Source: CAD feature listing. Evaluate the final solid. Frame: model axes, mm. Face numbers are marked on the shaded views. A direction names the side the tool comes from. Give positions to 0.01 mm unless a question says otherwise; leave off trailing zeros. Loops run counter-clockwise (first coordinate to the right, second up) from the corner with the lowest first, then second, coordinate; pieces in that order, holes last. Notation, with made-up numbers: (16, -4) -> (32, -4) arc R11 cw to (32, 17) -> close; hole circle Ø6 at (24.25, 49.5). An arc over 180 degrees is marked (long way). Answer as a JSON object with one key per item and string values. Group by question number.
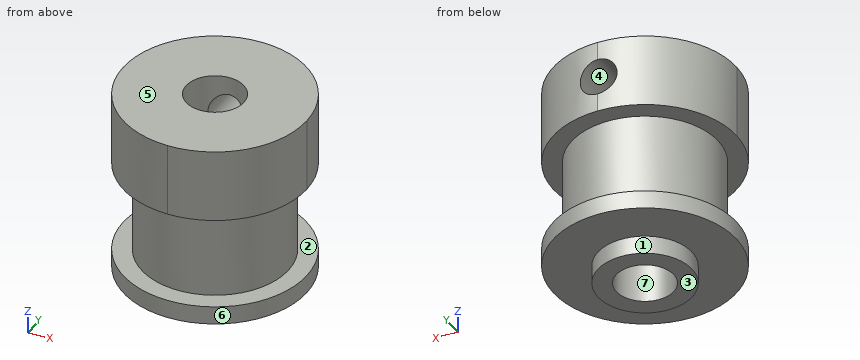
from build123d import *

# Parameters (mm, degrees)
F0_R         = 7.9375
F1_DEPTH     = 1.5875
F2_R         = 6.35
F3_DEPTH     = 8
F4_W         = 15.875
F4_H         = 15.875
F5_DEPTH     = 6.35
F6_R         = 2.5
F7_DEPTH     = 15.9375
F8_R         = 1.5875
F9_REACH     = 20.3661280605
F10_T1_DEPTH = 46.0375
F11_R        = 4.0875
F11_R_2      = 2.5
F12_DEPTH    = 1.5875


# Not quite as in the source:
# - a fillet or chamfer that OpenCascade refuses, or shapes differently, is made with other operations: its cross-section is extruded or revolved along the edge and cut away or added


with BuildPart() as f1:
    # F0 (on Top) → F1 (new body)
    with BuildSketch(Plane.XY):
        Circle(F0_R)
    extrude(amount=F1_DEPTH)

    # F2 (on face) → F3 (join)
    with BuildSketch(Plane.XY.offset(1.5875)):
        Circle(F2_R)
    extrude(amount=F3_DEPTH)

    # F4 (on face) → F5 (join)
    with BuildSketch(Plane.XY.offset(9.5875)):
        Rectangle(F4_W, F4_H)
    extrude(amount=F5_DEPTH)

    # F6 (on face) → F7 (cut, through all)
    with BuildSketch(Plane.XY.offset(15.9375)):
        Circle(F6_R)
    extrude(amount=-F7_DEPTH, mode=Mode.SUBTRACT)

    f9_end = f1.faces().sort_by_distance((-2.5, 0, 7.96875))[0]
    # F8 (on face) → F9 (cut, up to a face of the model that its end follows)
    with BuildSketch(Plane(origin=(0, 7.9375, 0), x_dir=(-1, 0, 0), z_dir=(0, 1, 0))):
        with Locations((0, 12.7625)):
            Circle(F8_R)
    f9_long = extrude(amount=-F9_REACH, mode=Mode.PRIVATE)
    add(split(f9_long, bisect_by=f9_end, keep=Keep.ALL, mode=Mode.PRIVATE).solids().sort_by_distance((0, 7.9375, 12.7625))[0], mode=Mode.SUBTRACT)

    # F10: fillet of radius 7.9375 on 4 edges, made by hand

    # F10_s2 → F10_t1 (cut)
    with BuildSketch(Plane.XY.offset(-10.25625)):
        with BuildLine():
            ThreePointArc((-7.9375, 0), (-5.6126600757, 5.6126600757), (0, 7.9375))
            Line((0, 7.9375), (-7.9375, 7.9375))
            Line((-7.9375, 7.9375), (-7.9375, 0))
        make_face()
        with BuildLine():
            ThreePointArc((0, -7.9375), (-5.6126600757, -5.6126600757), (-7.9375, 0))
            Line((-7.9375, 0), (-7.9375, -7.9375))
            Line((-7.9375, -7.9375), (0, -7.9375))
        make_face()
        with BuildLine():
            ThreePointArc((7.9375, 0), (5.6126600757, 5.6126600757), (0, 7.9375))
            Line((0, 7.9375), (7.9375, 7.9375))
            Line((7.9375, 7.9375), (7.9375, 0))
        make_face()
        with BuildLine():
            ThreePointArc((0, -7.9375), (5.6126600757, -5.6126600757), (7.9375, 0))
            Line((7.9375, 0), (7.9375, -7.9375))
            Line((7.9375, -7.9375), (0, -7.9375))
        make_face()
    extrude(amount=F10_T1_DEPTH, mode=Mode.SUBTRACT)

    # F11 (on face) → F12 (join)
    with BuildSketch(Plane(origin=(0, 0, 0), x_dir=(1, 0, 0), z_dir=(0, 0, -1))):
        Circle(F11_R)
        Circle(F11_R_2, mode=Mode.SUBTRACT)
    extrude(amount=F12_DEPTH)


solid = f1.part
(1) Mould query, pull axis X, two halves, no side actions, for the marked faces 5, 6 and 7. Classes: pulls with the +X half, pulls with the -X half, needs draft (parallel to the pull), parting line crosses it, or undercut.
(2) First-contact query: pin 1 (1.5 mm diameter, centred on y = 0.5, z = 6.5, fed in from +X); pin 2 (8 mm diameter, centred on x = 5.5, z = 14, fed in from +Y); pin 3 (5 mm diameter, centred on y = 5, z = 3.5, fed in from +X). Flat tips, straight axial feed; report the tip coordinate or a pass-through.
(3) Section query C-C on z = 3.25. Return the cut outline in (x, y), plus the area to 3 significant figures.
(4) Section query A-A on x = 2. Return the cut outline in (y, z), plus the area to 3 significant figures.
(5) Access query for the marked faces 1, 2, 3 and 4. Directions: +Z, -Z, +X, -X, +Y, -Y. A direction counts if a zero-diameter tool reaches every point of the face in a straight line with its end or side. Return the directions, or none.
(6) Section query D-D on x = -5.75. Return the cut outline in (y, z), plus the area to 3 significant figures.
(7) Section query B-B on y = 1.5. Return the cut outline in (x, z), plus the area to 3 significant figures.
(8) Material intervals for line 1 (Y direction, x = 0, z = 1); line 2 (Y direction, x = 0, z = 8); line 3 (X direction, y = 4.25, z = 13), sorted ascending. Write a range as from..to.
Result:
{
 "1": {"face 5": "needs draft", "face 6": "parting line crosses it", "face 7": "undercut"},
 "2": {"pin 1": "x = 6.35", "pin 2": "y = 7.79", "pin 3": "x = 7.18"},
 "3": {"outline": "circle Ø12.7 at (0, 0); hole circle Ø5 at (0, 0)", "area": "107 mm²"},
 "4": {"outline": "(-7.68, 0) -> (-3.56, 0) -> (-3.56, -1.59) -> (-1.5, -1.59) -> (-1.5, 15.94) -> (-7.68, 15.94) -> (-7.68, 9.59) -> (-6.03, 9.59) -> (-6.03, 1.59) -> (-7.68, 1.59) -> close; (1.5, -1.59) -> (3.56, -1.59) -> (3.56, 0) -> (7.68, 0) -> (7.68, 1.59) -> (6.03, 1.59) -> (6.03, 9.59) -> (7.68, 9.59) -> (7.68, 15.94) -> (1.5, 15.94) -> close", "area": "177 mm²"},
 "5": {"face 1": "-Z", "face 2": "none", "face 3": "-Z, +X, -X, +Y, -Y", "face 4": "+Y"},
 "6": {"outline": "(-5.47, 0) -> (5.47, 0) -> (5.47, 1.59) -> (2.69, 1.59) -> (2.69, 9.59) -> (5.47, 9.59) -> (5.47, 15.94) -> (-5.47, 15.94) -> (-5.47, 9.59) -> (-2.69, 9.59) -> (-2.69, 1.59) -> (-5.47, 1.59) -> close", "area": "130 mm²"},
 "7": {"outline": "(-7.79, 0) -> (-3.8, 0) -> (-3.8, -1.59) -> (-2, -1.59) -> (-2, 15.94) -> (-7.79, 15.94) -> (-7.79, 9.59) -> (-6.17, 9.59) -> (-6.17, 1.59) -> (-7.79, 1.59) -> close; (2, -1.59) -> (3.8, -1.59) -> (3.8, 0) -> (7.79, 0) -> (7.79, 1.59) -> (6.17, 1.59) -> (6.17, 9.59) -> (7.79, 9.59) -> (7.79, 15.94) -> (2, 15.94) -> close", "area": "164 mm²"},
 "8": {"line 1": "-7.94..-2.5, 2.5..7.94", "line 2": "-6.35..-2.5, 2.5..6.35", "line 3": "-6.7..-1.57, 1.57..6.7"}
}
